Source: CAD feature listing. Evaluate the final solid. Frame: model axes, mm. Give positions to 0.01 mm unless a question says otherwise; leave off trailing zeros. Write each loop counter-clockwise with the first axis right and the second up, starting at its lowest first coordinate (ties: lowest second). Pieces come first, ordered by that corner, then holes. Notation, with made-up numbers: (28.25, 18.25) - (42.25, 18.25) arc R8 ccw to (42.25, 30.25) - close; hole circle Ø2 at (-8, -23). An arc over 180 degrees is marked (long way). One line per question, with ' | ' between items. Start each with the question number.
(1) Pin query (flat end, axial travel): pin 1 (4.5 mm diameter, centred on x = -15, y = 12.5, fed in from -Z). Return the tip coordinate at first contact, or that it passes through.
(2) Ray query, line 1 (X direction, y = -4, z = 0.9); line 2 (Y direction, x = 4.5, z = 0.45); line 3 (Y direction, x = -13.5, z = 0.6). Return the intervals inside material, ascending. Write a range as [from, to].
(3) Section B-B, the plane y = -3. Return loops of the section in (x, z).
(4) Section C-C, the plane x = 5.5. Return loops of the section in (y, z).
(5) Section D-D, the plane y = -12. Return loops of the section in (x, z), plus the area to 3 significant figures.
(6) Section A-A, the plane z = 1.05. Return loops of the section in (x, y) (3 decimals).
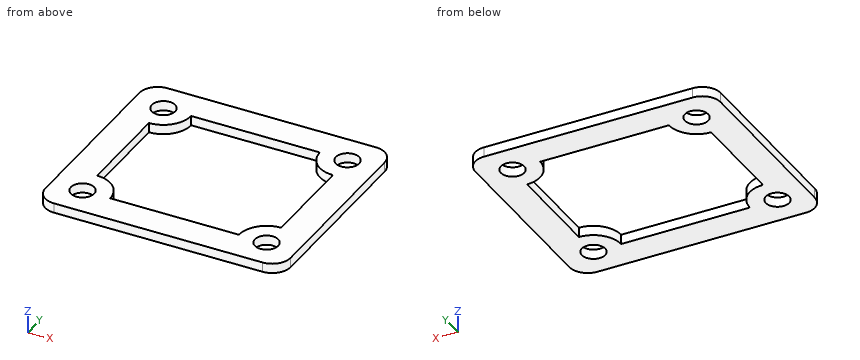
```python
from build123d import *

# Parameters (mm, degrees)
SKETCH1_W           = 40
SKETCH1_H           = 35
SKETCH1_R           = 1.905
BOSS_EXTRUDE1_DEPTH = 1.5875
FILLET1_R           = 3


with BuildPart() as part:
    # Sketch1 → Boss-Extrude1 (new body)
    with BuildSketch(Plane.XY):
        Rectangle(SKETCH1_W, SKETCH1_H)
        with Locations((-15, -12.5)):
            Circle(SKETCH1_R, mode=Mode.SUBTRACT)
        with Locations(Location((15, -12.5, 0), (0, 0, 180))):
            Circle(SKETCH1_R, mode=Mode.SUBTRACT)
        with Locations((15, 12.5)):
            Circle(SKETCH1_R, mode=Mode.SUBTRACT)
        with Locations(Location((-15, 12.5, 0), (0, 0, 180))):
            Circle(SKETCH1_R, mode=Mode.SUBTRACT)
        with BuildLine():
            Line((-15, 8), (-15, -8))
            ThreePointArc((-15, -8), (-11.818019485, -9.318019485), (-10.5, -12.5))
            Line((-10.5, -12.5), (10.5, -12.5))
            ThreePointArc((10.5, -12.5), (11.818019485, -9.318019485), (15, -8))
            Line((15, -8), (15, 8))
            ThreePointArc((15, 8), (11.818019485, 9.318019485), (10.5, 12.5))
            Line((10.5, 12.5), (-10.5, 12.5))
            ThreePointArc((-10.5, 12.5), (-11.818019485, 9.318019485), (-15, 8))
        make_face(mode=Mode.SUBTRACT)
    extrude(amount=BOSS_EXTRUDE1_DEPTH)

    # Fillet1
    fillet1_edges = [part.edges().sort_by_distance(p)[0] for p in [
        (20, -17.5, 0.79375),
        (-20, -17.5, 0.79375),
        (-20, 17.5, 0.79375),
        (20, 17.5, 0.79375),
    ]]
    fillet(fillet1_edges, radius=FILLET1_R)


solid = part.part
```
Check sheet entries:
1) pin 1: z = 0
2) line 1: [-20, -15], [15, 20] | line 2: [-17.5, -12.5], [12.5, 17.5] | line 3: [-17.5, -13.67], [-11.33, -8.26], [8.26, 11.33], [13.67, 17.5]
3) outline: (-20, 0) - (-15, 0) - (-15, 1.59) - (-20, 1.59) - close; (15, 0) - (20, 0) - (20, 1.59) - (15, 1.59) - close
4) outline: (-17.5, 0) - (-12.5, 0) - (-12.5, 1.59) - (-17.5, 1.59) - close; (12.5, 0) - (17.5, 0) - (17.5, 1.59) - (12.5, 1.59) - close
5) outline: (-20, 0) - (-16.84, 0) - (-16.84, 1.59) - (-20, 1.59) - close; (-13.16, 0) - (-10.53, 0) - (-10.53, 1.59) - (-13.16, 1.59) - close; (10.53, 0) - (13.16, 0) - (13.16, 1.59) - (10.53, 1.59) - close; (16.84, 0) - (20, 0) - (20, 1.59) - (16.84, 1.59) - close | area: 18.4 mm²
6) outline: (-20, -14.5) arc R3 ccw to (-17, -17.5) - (17, -17.5) arc R3 ccw to (20, -14.5) - (20, 14.5) arc R3 ccw to (17, 17.5) - (-17, 17.5) arc R3 ccw to (-20, 14.5) - close; hole circle Ø3.81 at (-15, -12.5); hole circle Ø3.81 at (-15, 12.5); hole (-15, -8) arc R4.5 cw to (-10.5, -12.5) - (10.5, -12.5) arc R4.5 cw to (15, -8) - (15, 8) arc R4.5 cw to (10.5, 12.5) - (-10.5, 12.5) arc R4.5 cw to (-15, 8) - close; hole circle Ø3.81 at (15, -12.5); hole circle Ø3.81 at (15, 12.5)
